Geometry: see drawing. Coordinates: mm, zero at the bounding-box minimum. A direction names the side the tool comes from. Coordinates: 2 decimals unless noted, no trailing zeros. Loops run counter-clockwise (first coordinate to the right, second up) from the corner with the lowest first, then second, coordinate; pieces in that order, holes last. Notation, with made-up numbers: (-1.5, -27) - (28.5, -27) arc R23 ccw to (28.5, 3) - close; hole circle Ø6 at (-39.5, 59.5). An arc over 180 degrees is marked (long way). Use one line per item in the form item = value.
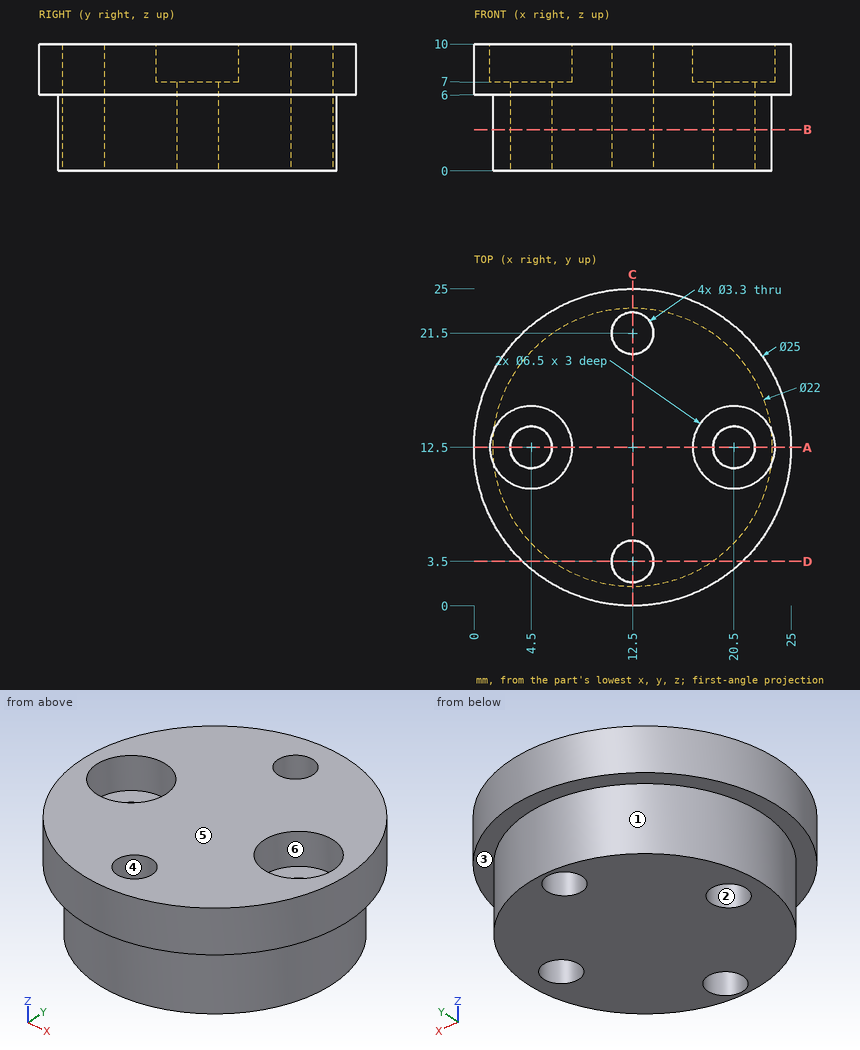
Q1. Cut plane D-D, the plane y = 3.5. Return loops of the section in (x, z), then the cut area to 3 significant figures.
Check values:
outline = (3.83, 6) - (6.18, 6) - (6.18, 0) - (10.85, 0) - (10.85, 10) - (3.83, 10) - close; (14.15, 0) - (18.82, 0) - (18.82, 6) - (21.17, 6) - (21.17, 10) - (14.15, 10) - close
area = 112 mm²
Q2. First-contact query: P1, Ø2, axis at x = 18.5, y = 13, coming from the +Z side; P2, Ø1, axis at x = 3, z = 7.5, coming from the -Y side; P3, Ø1.5, axis at x = 6.5, z = 6.5, coming from the -Y side. Flat tips, straight axial feed; report the tip coordinate or a pass-through.
Check values:
P1 = 7
P2 = 3.83
P3 = 1.16
Q3. Pull-direction query (Y, two-part tool) for the marked faces 1, 2, 3 and 4; classes: pulls with the +Y half, pulls with the -Y half, needs draft (parallel to the pull), parting line crosses it, or undercut.
Check values:
face_1 = parting line crosses it
face_2 = undercut
face_3 = needs draft
face_4 = undercut
Q4. Cut plane A-A, the plane y = 12.5. Return loops of the section in (x, z).
Check values:
outline = (0, 6) - (1.5, 6) - (1.5, 0) - (2.85, 0) - (2.85, 7) - (1.25, 7) - (1.25, 10) - (0, 10) - close; (6.15, 0) - (18.85, 0) - (18.85, 7) - (17.25, 7) - (17.25, 10) - (7.75, 10) - (7.75, 7) - (6.15, 7) - close; (22.15, 0) - (23.5, 0) - (23.5, 6) - (25, 6) - (25, 10) - (23.75, 10) - (23.75, 7) - (22.15, 7) - close
Q5. Ray query, line 1 along Y through (x, z) = (12.5, 4.25); line 2 along X through (y, z) = (12.25, 7.5); line 3 along Z through (x, y) = (17.75, 22.5). Return the intervals inside material, ascending. Write a range as [from, to].
Check values:
line_1 = [1.5, 1.85], [5.15, 19.85], [23.15, 23.5]
line_2 = [0, 1.26], [7.74, 17.26], [23.74, 25]
line_3 = [6, 10]
Q6. Set-up query: the marked faces 5 and 6. Return all of +Z, -Z, +X, -X, +Y, -Y with unobstructed straight access to the full face (end or side cutting, diameter ignored); none if empty.
Check values:
face_5 = +Z, +X, -X, +Y, -Y
face_6 = +Z
Q7. Cut plane B-B, the plane z = 3.25. Return loops of the section in (x, y), then the cut area to 3 significant figures.
Check values:
outline = circle Ø22 at (12.5, 12.5); hole circle Ø3.3 at (4.5, 12.5); hole circle Ø3.3 at (12.5, 3.5); hole circle Ø3.3 at (12.5, 21.5); hole circle Ø3.3 at (20.5, 12.5)
area = 346 mm²
Q8. Cut plane C-C, the plane x = 12.5. Return loops of the section in (y, z).
Check values:
outline = (0, 6) - (1.5, 6) - (1.5, 0) - (1.85, 0) - (1.85, 10) - (0, 10) - close; (5.15, 0) - (19.85, 0) - (19.85, 10) - (5.15, 10) - close; (23.15, 0) - (23.5, 0) - (23.5, 6) - (25, 6) - (25, 10) - (23.15, 10) - close
